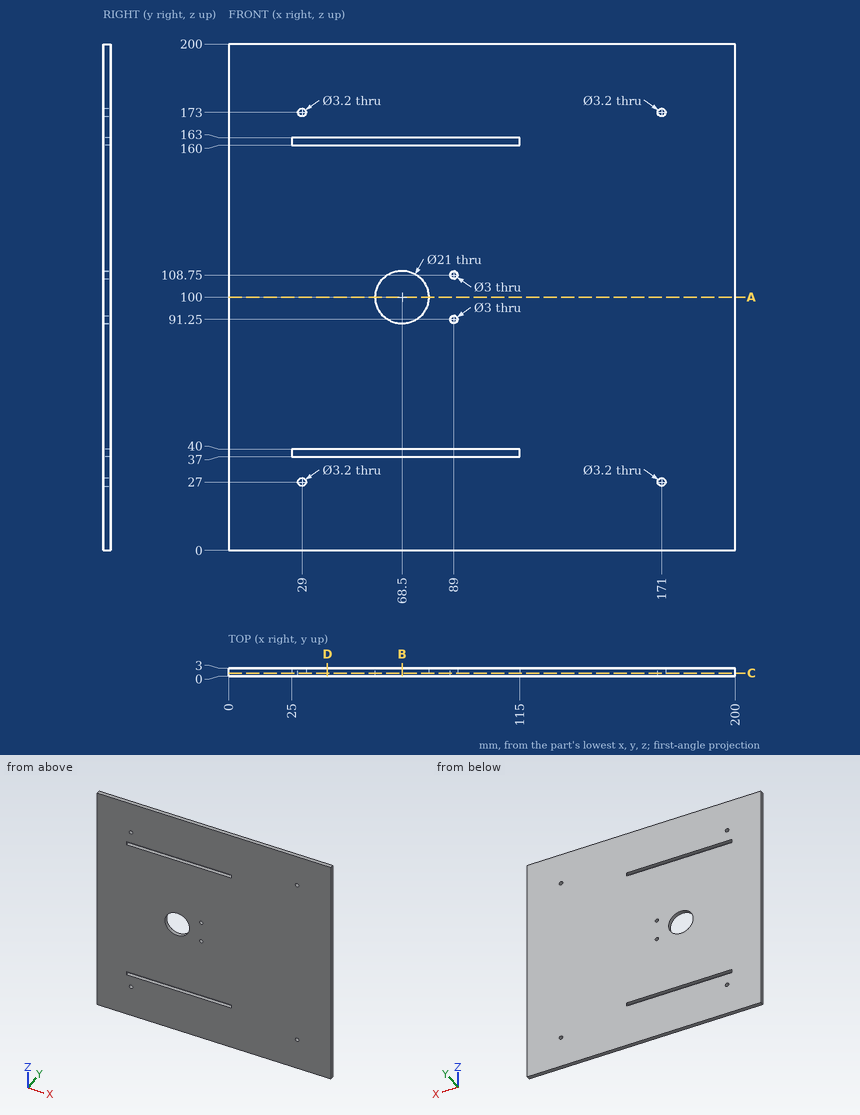
Study the drawing (mm; zero at the part's minimum x, y, z) and answer. Round coordinates to 2 decimals unless told otherwise and drop trailing zeros. Write each loop counter-clockwise with the first axis right and the second up, starting at its lowest first coordinate (ties: lowest second). Pieces come first, ordered by that corner, then holes. Notation, with made-up numbers: (25, 13.5) -> (55, 13.5) arc R11 cw to (55, 23.5) -> close; hole circle Ø9 at (29.5, -20). An arc over 180 degrees is marked (long way). Write item = value, one per line.
1) Straight lines are drawn through the part: line 1 along Z through (x, y) = (89, 0.7); line 2 along Z through (x, y) = (66.5, 1.7); line 3 along Z through (x, y) = (69.5, 2.9). For each, find the intervals that lie inside material, in ascending order. Write a range as [from, to].
Check values:
line_1 = [0, 37], [40, 89.75], [92.75, 107.25], [110.25, 160], [163, 200]
line_2 = [0, 37], [40, 89.69], [110.31, 160], [163, 200]
line_3 = [0, 37], [40, 89.55], [110.45, 160], [163, 200]
2) Section B-B on x = 68.5 is taken. Write down the section's boundary in (y, z), plus the area to 3 significant figures.
Check values:
outline = (0, 0) -> (3, 0) -> (3, 37) -> (0, 37) -> close; (0, 40) -> (3, 40) -> (3, 89.5) -> (0, 89.5) -> close; (0, 110.5) -> (3, 110.5) -> (3, 160) -> (0, 160) -> close; (0, 163) -> (3, 163) -> (3, 200) -> (0, 200) -> close
area = 519 mm²
3) Section A-A on z = 100 is taken. Write down the section's boundary in (x, y), plus the area to 3 significant figures.
Check values:
outline = (0, 0) -> (58, 0) -> (58, 3) -> (0, 3) -> close; (79, 0) -> (200, 0) -> (200, 3) -> (79, 3) -> close
area = 537 mm²
4) Section D-D on x = 39 is taken. Write down the section's boundary in (y, z), plus the area to 3 significant figures.
Check values:
outline = (0, 0) -> (3, 0) -> (3, 37) -> (0, 37) -> close; (0, 40) -> (3, 40) -> (3, 160) -> (0, 160) -> close; (0, 163) -> (3, 163) -> (3, 200) -> (0, 200) -> close
area = 582 mm²
5) Section C-C on y = 1.1 is taken. Give the number of separate pieces and of enclosed holes in the cut face, plus the area to 3 significant figures.
Check values:
separate_pieces = 1
enclosed_holes = 9
area = 39,100 mm²
6) Given pin 1 (3 mm diameter, centred on x = 171, z = 173, fed in from +Y), flat-ended and moving along its own axis, determine where the tip first touches the part or whether it passes through.
Check values:
pin_1 = through
